Could you check a few things on this model? Use its own coordinates, in mm. Face numbers are marked on the shaded views. Give positions to 0.01 mm unless a question says otherwise; leave off trailing zeros. Order: outer loops, then holes, each group sorted by start corner. A loop starts at its lowest first (then second) coordinate and runs counter-clockwise, first axis right, second up. Notation, with made-up numbers: M -32,53.5 L -14,53.5 A17 ccw -14,81.5 Z; hole C -0.5,-7.5 d1. An arc over 180 degrees is marked long. Use a Markdown table: item, result. Add a question column.
Item 1: Suppose I cut it at A-A on x = 24. Write out the boundary of the cut face in (y, z).
Item 2: I'm going to push flat-ended pins straight in: pin 1 Ø5 at (x, z) = (-6.5, 12.5) entering from +Y; pin 2 Ø1.5 at (x, y) = (-26, 11) entering from +Z; pin 3 Ø4 at (x, z) = (20, 10) entering from -Y. Where does each tip first touch, or does it pass through?
Item 3: If I drill on L1, parallel to Z at x = -20, y = 8.3; L2, parallel to Y at x = -13, z = 15.25; L3, parallel to X at y = 2, z = 13, over which ranges is the centre line in solid material (lowest first)? Write a range as from..to.
Item 4: Suppose I cut it at D-D on x = -20. Write out the boundary of the cut face in (y, z).
Item 5: Suppose I cut it at B-B on z = 10. Write out the boundary of the cut face in (x, y).
Item 6: Suppose I cut it at C-C on z = 2. Write out the boundary of the cut face in (x, y).
Item 7: If we mould it in two halves opening along X, with no side actions, what happens to the marked faces 1, 2, 3 and 4? For each: released by +X, released by -X, zero draft, split by the parting line, or undercut.
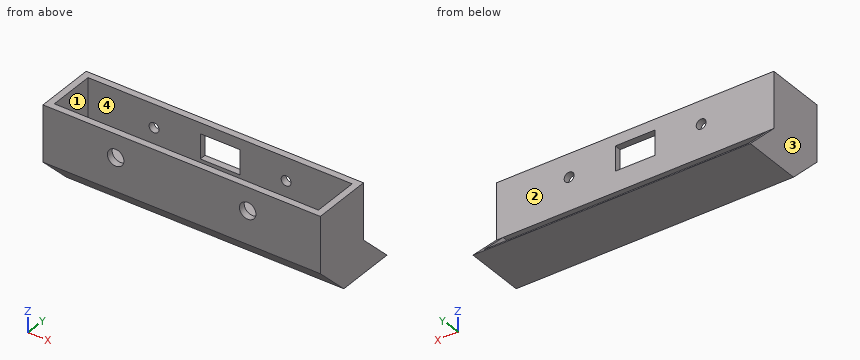
from build123d import *

# Parameters (mm, degrees)
F0_W           = 84
F0_H           = 18.2
F0_W_2         = 80
F0_H_2         = 14.2
F1_DEPTH       = 17
F3_D           = 3
F3_CBORE_D     = 5
F3_CBORE_DEPTH = 5
F4_W           = 12
F4_H           = 7.5
F5_DEPTH       = 2
F7_DEPTH       = 2
F9_DEPTH       = 2
F11_DEPTH      = 80
F13_DEPTH      = 80


with BuildPart() as f1:
    # F0 (on Top) → F1 (new body)
    with BuildSketch(Plane.XY):
        Rectangle(F0_W, F0_H)
        Rectangle(F0_W_2, F0_H_2, mode=Mode.SUBTRACT)
    extrude(amount=F1_DEPTH)

    # F3 (through all)
    with Locations(Plane.XZ.offset(9.1)):
        with Locations((-20, 10), (20, 10)):
            CounterBoreHole(F3_D / 2, F3_CBORE_D / 2, F3_CBORE_DEPTH)

    # F4 (on face) → F5 (cut)
    with BuildSketch(Plane(origin=(0, 9.1, 0), x_dir=(-1, 0, 0), z_dir=(0, 1, 0))):
        with Locations((0, 10)):
            Rectangle(F4_W, F4_H)
    extrude(amount=-F5_DEPTH, mode=Mode.SUBTRACT)

    # F6 (on face) → F7 (join)
    with BuildSketch(Plane(origin=(-42, 0, 0), x_dir=(0, -1, 0), z_dir=(-1, 0, 0))):
        Polygon((9.1, 0), (-9.1, 0), (-18.999495, -9.899495), (-0.799495, -9.899495), align=None)
    extrude(amount=-F7_DEPTH)

    # F8 (on face) → F9 (join)
    with BuildSketch(Plane.YZ.offset(42)):
        Polygon((9.1, 0), (-9.1, 0), (0.799495, -9.899495), (18.999495, -9.899495), align=None)
    extrude(amount=-F9_DEPTH)

    # F10 (on face) → F11 (join)
    with BuildSketch(Plane(origin=(40, 0, 0), x_dir=(0, -1, 0), z_dir=(-1, 0, 0))):
        Polygon((9.1, 0), (7.1, 0), (-2.799495, -9.899495), (-0.799495, -9.899495), align=None)
    extrude(amount=F11_DEPTH)

    # F12 (on face) → F13 (join)
    with BuildSketch(Plane(origin=(40, 0, 0), x_dir=(0, -1, 0), z_dir=(-1, 0, 0))):
        Polygon((-0.799495, -7.899495), (-16.999495, -7.899495), (-18.999495, -9.899495), (-2.799495, -9.899495), align=None)
    extrude(amount=F13_DEPTH)


solid = f1.part
Findings below:
| question | item | result |
|---|---|---|
| 1 | outline | M -9.1,0 L 0.8,-9.9 L 19,-9.9 L 17,-7.9 L 0.8,-7.9 L -7.1,0 L -7.1,17 L -9.1,17 Z; M 7.1,0 L 9.1,0 L 9.1,17 L 7.1,17 Z |
| 2 | pin 1 | stops at y = 9.1 |
| 2 | pin 2 | stops at z = -7.9 |
| 2 | pin 3 | stops at y = 7.1 |
| 3 | L1 | z = -9.9..-7.9, 0..8.5, 11.5..17 |
| 3 | L2 | y = -9.1..-7.1, 7.1..9.1 |
| 3 | L3 | x = -42..-40, 40..42 |
| 4 | outline | M -9.1,0 L 0.8,-9.9 L 19,-9.9 L 17,-7.9 L 0.8,-7.9 L -7.1,0 L -7.1,7.5 L -9.1,7.5 Z; M -9.1,12.5 L -7.1,12.5 L -7.1,17 L -9.1,17 Z; M 7.1,0 L 9.1,0 L 9.1,8.5 L 7.1,8.5 Z; M 7.1,11.5 L 9.1,11.5 L 9.1,17 L 7.1,17 Z |
| 5 | outline | M -42,-9.1 L -22.5,-9.1 L -22.5,-7.1 L -40,-7.1 L -40,7.1 L -21.5,7.1 L -21.5,9.1 L -42,9.1 Z; M -18.5,7.1 L -6,7.1 L -6,9.1 L -18.5,9.1 Z; M -17.5,-9.1 L 17.5,-9.1 L 17.5,-7.1 L -17.5,-7.1 Z; M 6,7.1 L 18.5,7.1 L 18.5,9.1 L 6,9.1 Z; M 21.5,7.1 L 40,7.1 L 40,-7.1 L 22.5,-7.1 L 22.5,-9.1 L 42,-9.1 L 42,9.1 L 21.5,9.1 Z |
| 6 | outline | M -42,-9.1 L 42,-9.1 L 42,9.1 L -42,9.1 Z; hole M -40,-7.1 L 40,-7.1 L 40,7.1 L -40,7.1 Z |
| 7 | face 1 | undercut |
| 7 | face 2 | zero draft |
| 7 | face 3 | released by -X |
| 7 | face 4 | undercut |
